Geometry: final body of the model. Coordinates: model frame, mm. A direction names the side the tool comes from. Give positions to 0.01 mm unless a question says otherwise; leave off trailing zeros. Order: outer loops, then holes, each group sorted by start corner. A loop starts at its lowest first (then second) coordinate and runs counter-clockwise, first axis right, second up. Notation, with made-up numbers: (45, -4.75) -> (83, -4.75) arc R32 ccw to (83, 28.25) -> close; hole circle Ø6 at (16.5, 17). An arc over 180 degrees is marked (long way). One line per item, written item: value. Start each with the question number.
```python
from build123d import *

# Parameters (mm, degrees)
F0_W     = 71.9074
F0_H     = 33.4264
F0_R     = 1.9812
F0_R_2   = 4.7752
F0_R_3   = 1.27
F1_DEPTH = 2.54
F3_DEPTH = 25.4
F4_W     = 35.56
F4_H     = 2.54
F5_DEPTH = 2.54
F7_DEPTH = 2.54
F8_R     = 3.4925
F8_R_2   = 1.27
F9_DEPTH = 2.159
F10_R    = 1.26999


# Not quite as in the source:
# - a fillet or chamfer is up to 0.001 mm smaller than in the source, because OpenCascade refuses the exact size


with BuildPart() as f1:
    # F0 (on Top) → F1 (new body)
    with BuildSketch(Plane.XY):
        with Locations((35.9537, 16.7132)):
            Rectangle(F0_W, F0_H)
        with Locations((26.1112, 9.5758)):
            Circle(F0_R, mode=Mode.SUBTRACT)
        with Locations((4.699, 17.5514)):
            Circle(F0_R, mode=Mode.SUBTRACT)
        with Locations((54.6862, 15.2908)):
            Circle(F0_R_2, mode=Mode.SUBTRACT)
        Polygon((71.9074, 0), (0, 0), (0, -1.0727777636), (0, -28.6960222364), (0, -32.6136), (71.9074, -32.6136), align=None)
        with Locations((3.6068, -14.8844)):
            Circle(F0_R_3, mode=Mode.SUBTRACT)
        with Locations((25.8572, -14.8844)):
            Circle(F0_R_3, mode=Mode.SUBTRACT)
        with BuildLine():
            Line((0, -28.6960222364), (0, -1.0727777636))
            ThreePointArc((0, -1.0727777636), (-10.668, -14.8844), (0, -28.6960222364))
        make_face()
    extrude(amount=F1_DEPTH)

    # F2 (on face) → F3 (cut)
    with BuildSketch(Plane.XY):
        with BuildLine():
            ThreePointArc((73.7104990378, 18.8731995366), (72.5573784353, 21.6570789342), (69.7734990378, 22.8101995366))
            Line((69.7734990378, 22.8101995366), (67.3858990378, 22.8101995366))
            ThreePointArc((67.3858990378, 22.8101995366), (64.6020196402, 21.6570789342), (63.4488990378, 18.8731995366))
            ThreePointArc((63.4488990378, 18.8731995366), (64.6020196402, 16.0893201391), (67.3858990378, 14.9361995366))
            Line((67.3858990378, 14.9361995366), (69.7734990378, 14.9361995366))
            ThreePointArc((69.7734990378, 14.9361995366), (72.5573784353, 16.0893201391), (73.7104990378, 18.8731995366))
        make_face()
        with BuildLine():
            ThreePointArc((45.7704990378, 18.8731995366), (44.6173784353, 21.6570789342), (41.8334990378, 22.8101995366))
            Line((41.8334990378, 22.8101995366), (39.4458990378, 22.8101995366))
            ThreePointArc((39.4458990378, 22.8101995366), (36.6620196402, 21.6570789342), (35.5088990378, 18.8731995366))
            ThreePointArc((35.5088990378, 18.8731995366), (36.6620196402, 16.0893201391), (39.4458990378, 14.9361995366))
            Line((39.4458990378, 14.9361995366), (41.8334990378, 14.9361995366))
            ThreePointArc((41.8334990378, 14.9361995366), (44.6173784353, 16.0893201391), (45.7704990378, 18.8731995366))
        make_face()
    extrude(amount=F3_DEPTH, mode=Mode.SUBTRACT)

    # F4 (on face) → F5 (join)
    with BuildSketch(Plane(origin=(0, 33.4264, 0), x_dir=(-1, 0, 0), z_dir=(0, 1, 0))):
        with Locations((-36.3474, 1.27)):
            Rectangle(F4_W, F4_H)
    extrude(amount=F5_DEPTH)

    # F6 (on face) → F7 (cut)
    with BuildSketch(Plane.XY.offset(2.54)):
        Polygon((18.5674, 33.4264), (21.1074, 33.4264), (18.5674, 35.9664), align=None)
        Polygon((54.1274, 33.4264), (54.1274, 35.9664), (51.5874, 33.4264), align=None)
    extrude(amount=-F7_DEPTH, mode=Mode.SUBTRACT)

    # F8 (on face) → F9 (cut)
    with BuildSketch(Plane.XY.offset(2.54)):
        with Locations((3.6068, -14.8844)):
            Circle(F8_R)
        with Locations((3.6068, -14.8844)):
            Circle(F8_R_2, mode=Mode.SUBTRACT)
        with Locations((25.8572, -14.8844)):
            Circle(F8_R)
        with Locations((25.8572, -14.8844)):
            Circle(F8_R_2, mode=Mode.SUBTRACT)
    extrude(amount=-F9_DEPTH, mode=Mode.SUBTRACT)

    # F10 (radius 1.27 in the source; OpenCascade refuses exactly that, so slightly less here)
    f10_edges = [f1.edges().sort_by_distance(p)[0] for p in [
        (35.508899, 18.8732, 2.54),
        (63.448899, 18.8732, 2.54),
        (63.448899, 18.8732, 0),
        (45.770499, 18.8732, 0),
    ]]
    fillet(f10_edges, radius=F10_R)


solid = f1.part
```
1. Cut plane A-A, the plane z = 1.95. Return loops of the section in (x, y) (1 decimal).
2. Material intervals for L1, parallel to X at y = 11, z = 2.15; L2, parallel to X at y = -18, z = 2.2; L3, parallel to X at y = 30.5, z = 0.7, sorted ascending. Write a range as [from, to].
3. Cut plane C-C, the plane y = 2.5. Return loops of the section in (x, z), then the cut area to 3 significant figures.
4. Access query for faces 1 (the cylindrical face through (-10.666, -14.622, 1.252)), 2 (the cylindrical face through (2.85, -18.294, 1.476)), 3 (the flat face through (0, 16, 1)). Directions: +Z, -Z, +X, -X, +Y, -Y. A direction counts if a zero-diameter tool reaches every point of the face in a straight line with its end or side. Return the directions, or none.
5. Draft query along Y for faces 4 (the flat face through (35, -32.614, 1)), 5 (the flat face through (0, -31, 1)), 6 (the cylindrical face through (28, 10.17, 1.25)). Return one class per face: pulls with the +Y half, pulls with the -Y half, needs draft (parallel to the pull), parting line crosses it, or undercut.
6. Pin query (flat end, axial travel): P1, Ø3.5, axis at x = 4.5, y = -14.5, coming from the +Z side; P2, Ø0.8, axis at x = 15.5, z = 2, coming from the +Y side. Return the tip coordinate at first contact, or that it passes through.
7. Cut plane B-B, the plane x = 12. Return loops of the section in (y, z).
Answers follow:
1. outline: (0, -32.6) -> (71.9, -32.6) -> (71.9, 15.3) arc R4.1 cw to (69.8, 14.7) -> (67.4, 14.7) arc R4.1 cw to (67.4, 23) -> (69.8, 23) arc R4.1 cw to (71.9, 22.4) -> (71.9, 33.4) -> (51.6, 33.4) -> (54.1, 36) -> (18.6, 36) -> (21.1, 33.4) -> (0, 33.4) -> (0, -1.1) arc R14.3 ccw to (0, -28.7) -> close; hole circle Ø7 at (3.6, -14.9); hole circle Ø4 at (4.7, 17.6); hole circle Ø7 at (25.9, -14.9); hole circle Ø4 at (26.1, 9.6); hole (39.4, 14.7) -> (41.8, 14.7) arc R4.1 ccw to (41.8, 23) -> (39.4, 23) arc R4.1 ccw to start; hole circle Ø9.6 at (54.7, 15.3)
2. L1: x = [0, 24.73], [27.49, 52.59], [56.78, 71.91]
2. L2: x = [-10.32, 2.03], [5.18, 24.28], [27.44, 71.91]
2. L3: x = [0, 71.91]
3. outline: (0, 0) -> (71.91, 0) -> (71.91, 2.54) -> (0, 2.54) -> close
3. area: 183 mm²
4. face 1: +Z, -Z, -X
4. face 2: +Z
4. face 3: +Z, -Z, -X, +Y
5. face 4: pulls with the -Y half
5. face 5: needs draft
5. face 6: undercut
6. P1: stops at z = 0.38
6. P2: stops at y = 33.43
7. outline: (-32.61, 0) -> (33.43, 0) -> (33.43, 2.54) -> (-32.61, 2.54) -> close
